The listing builds one solid part. Answer for the finished solid, in the listing's coordinates (mm). A direction names the side the tool comes from. Round coordinates to 2 decimals unless told otherwise and drop trailing zeros. Order: outer loops, then holes, each group sorted by start corner. A loop starts at its lowest first (then second) coordinate and runs counter-clockwise, first axis right, second up. Notation, with made-up numbers: (-12.75, -26.5) -> (35.25, -26.5) arc R23 ccw to (35.25, -10.5) -> close; hole circle Ø5 at (43, 81). An arc over 180 degrees is marked (long way). Answer in a Markdown table with one row per item. Add a question column.
```python
from build123d import *

# Parameters (mm, degrees)
F2_R     = 2.5
F3_DEPTH = 50.001


with BuildPart() as f1:
    # F0 (on Front) → F1 (revolve)
    with BuildSketch(Plane.XZ):
        Polygon((0, 50), (0, 0), (12.5, 0), (12.5, 1.2), (7.5, 1.2), (7.5, 3.422222), (12.5, 3.422222), (12.5, 4.622222), (7.5, 4.622222), (7.5, 6.844444), (12.5, 6.844444), (12.5, 8.044444), (7.5, 8.044444), (7.5, 10.266667), (12.5, 10.266667), (12.5, 11.466667), (7.5, 11.466667), (7.5, 13.688889), (12.5, 13.688889), (12.5, 14.888889), (7.5, 14.888889), (7.5, 17.111111), (12.5, 17.111111), (12.5, 18.311111), (7.5, 18.311111), (7.5, 20.533333), (12.5, 20.533333), (12.5, 21.733333), (7.5, 21.733333), (7.5, 23.955556), (12.5, 23.955556), (12.5, 25.155556), (7.5, 25.155556), (7.5, 27.377778), (12.5, 27.377778), (12.5, 28.577778), (7.5, 28.577778), (7.5, 30.8), (12.5, 30.8), (12.5, 32), (6, 32), (6, 34.3), (8, 34.3), (8, 35.5), (6, 35.5), (6, 38), (8, 38), (8, 41), (6, 41), (6, 45.8), (8, 45.8), (8, 50), align=None)
    revolve(axis=Axis((0, 0, 25), (0, 0, -1)))

    # F2 (on face) → F3 (cut, through all)
    with BuildSketch(Plane(origin=(0, 0, 0), x_dir=(1, 0, 0), z_dir=(0, 0, -1))):
        Circle(F2_R)
    extrude(amount=-F3_DEPTH, mode=Mode.SUBTRACT)


solid = f1.part
```
1. Each of these flat-tipped pins is pushed along its axis until it touches: pin 1 (1.5 mm diameter, centred on y = 8, z = 5, fed in from +X); pin 2 (5 mm diameter, centred on y = -1, z = 40, fed in from -X); pin 3 (3 mm diameter, centred on x = 2, z = 9, fed in from +Y). Where does it stop, or does it pass through?
2. The part is cut by section B-B (y = -9). Give the number of separate pieces and of enclosed holes in the cut face, then the cut area to 3 significant figures.
3. Straight lines are drawn through the part: line 1 along Z through (x, y) = (6.25, -1.25); line 2 along X through (y, z) = (0, 30); line 3 along X through (y, z) = (0, 35). For each, find the intervals that lie inside material, in ascending order.
4. The mould has two halves that part along X. Classify faces 1 (the cylindrical face through (11.923, -3.755, 24.564)), 2 (the cylindrical face through (-0.54, 2.44, 24.65)), 3 (the flat face through (-2, -6, 35.5)): released by +X, released by -X, zero draft, split by the parting line, or undercut.
5. The part is cut by section A-A (z = 15.5). Give the vertices of the cut face in (x, y), then the cut area to 3 significant figures.
6. For faces 4 (the flat face through (-3, 5.4, 32)), 5 (the cylindrical face through (-1.73, 7.81, 39.52)), 6 (the cylindrical face through (11.923, -3.755, 10.875)), determine the directions among +Z, -Z, +X, -X, +Y, -Y from which every point of the face is accessible in a straight line to the end or side of a thin tool.
Report:
| question | item | result |
|---|---|---|
| 1 | pin 1 | stops at x = 10.11 |
| 1 | pin 2 | stops at x = -8 |
| 1 | pin 3 | stops at y = 12.47 |
| 2 | separate pieces | 10 |
| 2 | enclosed holes | 0 |
| 2 | area | 208 mm^2 |
| 3 | line 1 | z = 0 to 32, 34.3 to 35.5, 38 to 41, 45.8 to 50 |
| 3 | line 2 | x = -7.5 to -2.5, 2.5 to 7.5 |
| 3 | line 3 | x = -8 to -2.5, 2.5 to 8 |
| 4 | face 1 | split by the parting line |
| 4 | face 2 | undercut |
| 4 | face 3 | zero draft |
| 5 | outline | circle Ø15 at (0, 0); hole circle Ø5 at (0, 0) |
| 5 | area | 157 mm^2 |
| 6 | face 4 | none |
| 6 | face 5 | +Z |
| 6 | face 6 | +Z, -Z |
